Verification items for the finished model (mm, model axes). A direction names the side the tool comes from. Give positions to 0.01 mm unless a question says otherwise; leave off trailing zeros. Loops run counter-clockwise (first coordinate to the right, second up) from the corner with the lowest first, then second, coordinate; pieces in that order, holes last. Notation, with made-up numbers: (37.25, -30.5) - (66.25, -30.5) arc R18 ccw to (66.25, -22.5) - close; hole circle Ø10 at (29, -36). An arc over 180 degrees is marked (long way). One line per item, written item: value. Start each with the question number.
1. Sectioned sample at B-B (y = 91.5). Record the cut outline in (x, z), plus the area to 3 significant figures.
2. Sectioned sample at A-A (x = 92). Record the cut outline in (y, z).
3. Access from +Z, -Z, +X, -X, +Y, -Y to the whole of each face (thin tool, end or side, straight path). Record for faces 1 (the flat face through (155, 147, -3)), 2 (the flat face through (-165, 5, 74)).
4. Gauge pin test, flat ends, axial feed: pin 1 (6 mm diameter, centred on x = -88, y = 204.5, fed in from -Z); pin 2 (1 mm diameter, centred on y = 220, z = -26.5, fed in from -X). Record the tip position at first contact, or that the pin passes through.
5. Scan lines: L1, parallel to Y at x = 91, z = 134; L2, parallel to Z at x = -98, y = 172. Record each from-to range of solid material in increasing order. Write a range as [from, to].
Autodesk Inventor part; units mm, degrees
ref_plane "YZ Plane" through (0, 0, 0) normal (1, 0, 0) x (0, 1, 0)
ref_plane "XY Plane" through (0, 0, 0) normal (0, 0, 1) x (1, 0, 0)
sketch "Sketch1" plane through (0, 0, 0) normal (0, 1, 0) x (-1, 0, 0)
  line L0 (155, 155) -> (-155, 155)
  line L1 (-155, 155) -> (-155, -155)
  line L2 (-155, -155) -> (155, -155)
  line L3 (155, -155) -> (155, 155)
  line L4 (155, 155) -> (-155, -155) construction
  line L5 (-155, 155) -> (155, -155) construction
  line L6 (165, -165) -> (-165, -165)
  line L7 (-165, -165) -> (-165, 165)
  line L8 (-165, 165) -> (165, 165)
  line L9 (165, 165) -> (165, -165)
  point P0 (0, 0)
  dimension "d0" = 310
  dimension "d1" = 310
extrude "Extrusion1" add sketch "Sketch1" along normal blind 10 contours L3 L2 L1 L0 | L6 L7 L8 L9
extrude "Extrusion2" add sketch "Sketch1" along normal blind 280
sketch "Sketch4" plane through (0, 280, 0) normal (0, 1, 0) x (1, 0, 0)
  line L0 (-155, 155) -> (-155, -155)
  line L1 (-155, -155) -> (155, -155)
  line L2 (155, -155) -> (155, 155)
  line L3 (155, 155) -> (-155, 155)
  point P0 (0, 0)
  dimension "d6" = 310
  dimension "d7" = 310
sketch "Sketch5" plane through (155, 10, 155) normal (-1, 0, 0) x (0, 0, 1)
  line L0 (0, 0) -> (-310, 0)
  line L1 (0, 0) -> (0, 270)
  line L2 (-310, 270) -> (0, 270)
  line L3 (-310, 0) -> (-310, 270)
  point P0 (-155, -10)
  dimension "d8" = 270
sketch "Sketch6" plane through (0, 10, 0) normal (0, 1, 0) x (1, 0, 0)
  line L0 (-155, 155) -> (-155, -155)
  line L1 (-155, -155) -> (155, -155)
  line L2 (155, -155) -> (155, 155)
  line L3 (155, 155) -> (-155, 155)
  point P0 (0, 0)
sketch "Sketch7" plane through (-155, 10, -155) normal (1, 0, 0) x (0, 0, -1)
  line L0 (0, 0) -> (-310, 0)
  line L1 (0, 0) -> (0, 270)
  line L2 (-310, 270) -> (0, 270)
  line L3 (-310, 0) -> (-310, 270)
  point P0 (-155, -10)
sketch "Sketch8" plane through (0, 280, 0) normal (0, 1, 0) x (1, 0, 0)
  line L0 (165, 165) -> (-165, 165)
  line L1 (155, 155) -> (155, 165)
  line L2 (-165, 165) -> (165, 165)
  line L3 (-155, 155) -> (-155, 165)
  line L4 (155, 155) -> (-155, 155)
  point P0 (0, 0)
  dimension "d0" = 310
extrude "Extrusion3" cut sketch "Sketch8" against normal blind 270
sketch "Sketch9" plane through (0, 280, 0) normal (0, 1, 0) x (1, 0, 0)
  line L0 (-155, -155) -> (-155, 165)
  line L1 (-155, 165) -> (-165, 165)
  line L2 (-165, 165) -> (-165, -165)
  line L3 (-165, -165) -> (165, -165)
  line L4 (165, -165) -> (165, 165)
  line L5 (165, 165) -> (155, 165)
  line L6 (155, 165) -> (155, -155)
  line L7 (155, -155) -> (-155, -155)
  line L8 (-155, -155) -> (-165, -155)
  point P0 (0, 0)
extrude "Extrusion4" cut sketch "Sketch9" against normal blind 270 contours L8 L2 L1 L0
ref_plane "Work Plane1" through (0, 10, 0) normal (0, 1, 0) x (-1, 0, 0)
properties part number "Box Pengukuran"
Results are:
1. outline: (-165, 155) - (155, 155) - (155, -165) - (165, -165) - (165, 165) - (-165, 165) - close
1. area: 6,500 mm^2
2. outline: (0, -165) - (10, -165) - (10, 155) - (280, 155) - (280, 165) - (0, 165) - close
3. face 1: -Z, -X, +Y
3. face 2: +Z, -Z, -X, +Y, -Y
4. pin 1: stops at z = 155
4. pin 2: stops at x = 155
5. L1: y = [0, 10]
5. L2: z = [155, 165]
